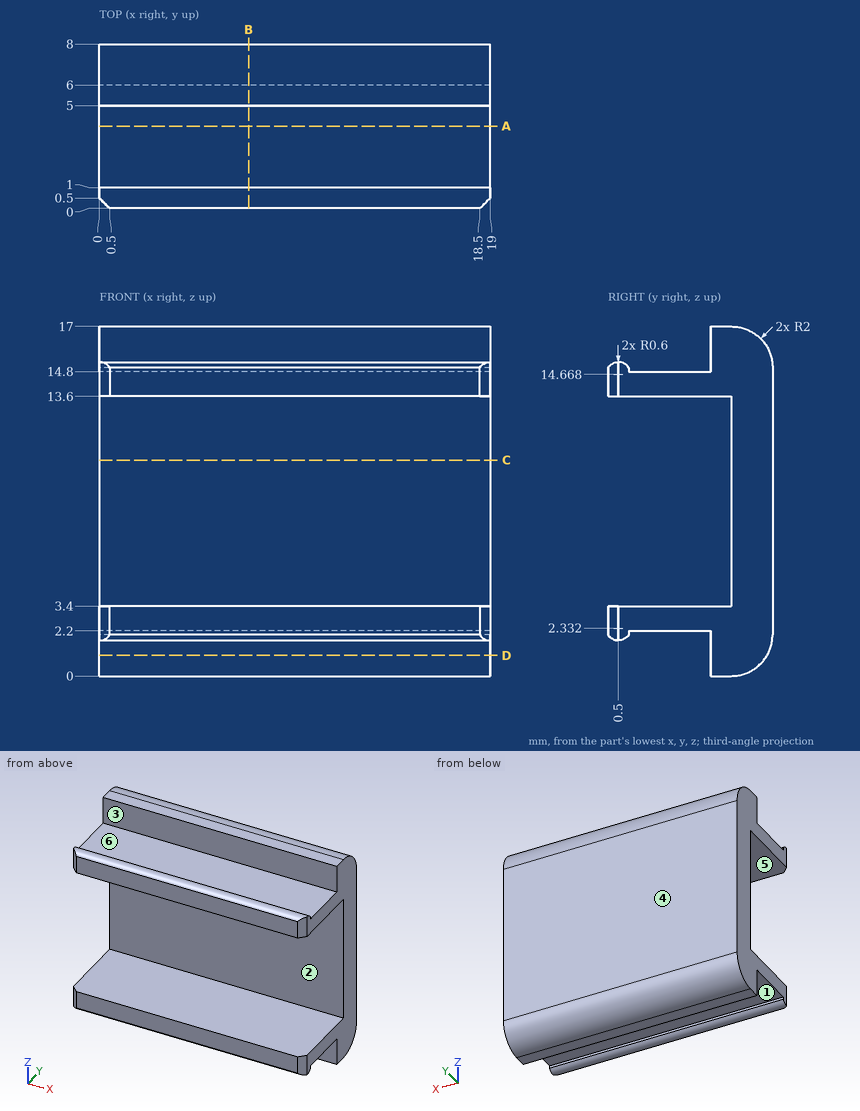
Check sheet for the drawn part. Datum: minimum x, y, z corner. Units: mm. A direction names the side the tool comes from. Round coordinates to 2 decimals unless told otherwise and drop trailing zeros. Loops run counter-clockwise (first coordinate to the right, second up) from the corner with the lowest first, then second, coordinate; pieces in that order, holes last. Notation, with made-up numbers: (63, 71.5) - (113, 71.5) arc R7 cw to (113, 80.5) - close; hole circle Ø10 at (-38, -14.75). An arc over 180 degrees is marked (long way). Answer as a JSON object with one key per item and string values. Group by question number.
Q1. Sectioned sample at A-A, the plane y = 4. Enter the section's corners in (x, z).
Q2. Mould release check, pull along Y, two halves, no side actions. Record for the marked faces 4, 5 and 6: released by +Y, released by -Y, zero draft, split by the parting line, or undercut.
Q3. Set-up check for the marked faces 1, 2 and 3: record each of +Z, -Z, +X, -X, +Y, -Y from which the full face is reachable in a straight line by a thin tool's end or side.
Q4. Sectioned sample at B-B, the plane x = 7.25. Enter the section's corners in (y, z).
Q5. Sectioned sample at D-D, the plane z = 1. Enter the section's corners in (x, y).
Q6. Sectioned sample at C-C, the plane z = 10.5. Enter the section's corners in (x, y), plus the area to 3 significant figures.
Q7. Gauge pin test, flat end, axial feed: P1, Ø3, axis at x = 10, y = 2, coming from the -Z side. Record the tip position at first contact, or that the pin passes through.
Q8. Scan lines: line 1 along Y through (x, z) = (8.5, 2); line 2 along Z through (x, y) = (15.5, 4.5); line 3 along Y through (x, z) = (11, 6.25). Record each from-to range of solid material in increasing order. Write a range as [from, to].
Solution:
{
 "1": {"outline": "(0, 2.2) - (19, 2.2) - (19, 3.4) - (0, 3.4) - close; (0, 13.6) - (19, 13.6) - (19, 14.8) - (0, 14.8) - close"},
 "2": {"face 4": "released by +Y", "face 5": "zero draft", "face 6": "undercut"},
 "3": {"face 1": "-Z, +X, -X", "face 2": "+X, -X, -Y", "face 3": "+Z, +X, -X"},
 "4": {"outline": "(0, 2) arc R0.6 ccw to (1, 2) - (1, 2.2) - (5, 2.2) - (5, 0) - (6, 0) arc R2 ccw to (8, 2) - (8, 15) arc R2 ccw to (6, 17) - (5, 17) - (5, 14.8) - (1, 14.8) - (1, 15) arc R0.6 ccw to (0, 15) - (0, 13.6) - (6, 13.6) - (6, 3.4) - (0, 3.4) - close"},
 "5": {"outline": "(0, 5) - (19, 5) - (19, 7.73) - (0, 7.73) - close"},
 "6": {"outline": "(0, 6) - (19, 6) - (19, 8) - (0, 8) - close", "area": "38.0 mm²"},
 "7": {"P1": "stops at z = 1.73"},
 "8": {"line 1": "y = [0, 1], [5, 8]", "line 2": "z = [2.2, 3.4], [13.6, 14.8]", "line 3": "y = [6, 8]"}
}
